Here's how the part is built. I have some questions about the finished solid (model axes, mm). Face numbers are marked on the shaded views. A direction names the side the tool comes from. Give positions to 0.01 mm unless a question says otherwise; leave off trailing zeros. Loops run counter-clockwise (first coordinate to the right, second up) from the corner with the lowest first, then second, coordinate; pieces in that order, holes last. Notation, with made-up numbers: (5, -4.5) - (42, -4.5) arc R14 cw to (42, 4.5) - close; hole circle Ø7 at (-40, 32.25). An arc over 180 degrees is marked (long way). Use one line per item in the form item = value.
from build123d import *

# Parameters (mm, degrees)
F0_R     = 1.795
F1_DEPTH = 3.1


with BuildPart() as f1:
    # F0 (on Front) → F1 (new body)
    with BuildSketch(Plane.XZ):
        with BuildLine():
            Line((-25.917618, 55.021677), (-33.917618, 50.898571))
            Line((-33.917618, 50.898571), (-33.917618, 30.898571))
            Line((-33.917618, 30.898571), (-26.205678, 16.406338))
            ThreePointArc((-26.205678, 16.406338), (-25.480558, 16.083714), (-24.99199, 16.709162))
            Line((-24.99199, 16.709162), (-24.99199, 34.125582))
            Line((-24.99199, 34.125582), (-28.417245, 37.768057))
            Line((-28.417245, 37.768057), (-28.417245, 42.768057))
            Line((-28.417245, 42.768057), (-22.746045, 37.125585))
            Line((-22.746045, 37.125585), (-22.746045, 24.125582))
            Line((-22.746045, 24.125582), (-20.271171, 21.650708))
            ThreePointArc((-20.271171, 21.650708), (-19.917618, 21.504262), (-19.564064, 21.650708))
            Line((-19.564064, 21.650708), (-17.089191, 24.125582))
            Line((-17.089191, 24.125582), (-17.089191, 37.125585))
            Line((-17.089191, 37.125585), (-11.41799, 42.768057))
            Line((-11.41799, 42.768057), (-11.41799, 37.768057))
            Line((-11.41799, 37.768057), (-14.843246, 34.125582))
            Line((-14.843246, 34.125582), (-14.843246, 16.690635))
            ThreePointArc((-14.843246, 16.690635), (-14.358181, 16.069672), (-13.638261, 16.389983))
            Line((-13.638261, 16.389983), (-5.917618, 30.898571))
            Line((-5.917618, 30.898571), (-5.917618, 50.898571))
            Line((-5.917618, 50.898571), (-13.917618, 55.021677))
            Line((-13.917618, 55.021677), (-25.917618, 55.021677))
        make_face()
        with Locations((-20.491593, 51.844455)):
            Circle(F0_R, mode=Mode.SUBTRACT)
    extrude(amount=F1_DEPTH)


solid = f1.part
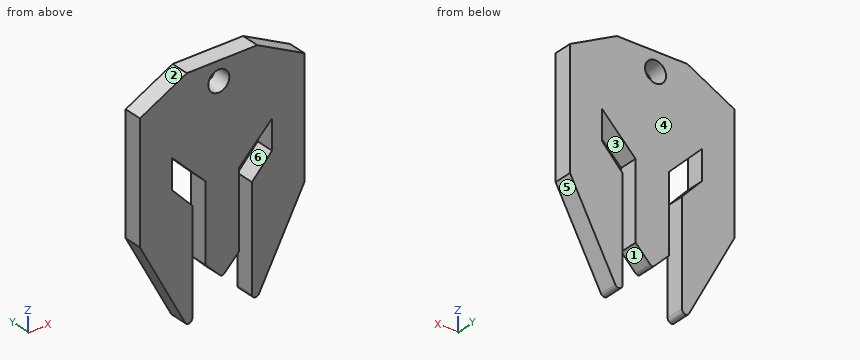
(1) For P1, Ø1, axis at x = -10.5, y = -1.5, coming from the -Z side; P2, Ø0.9, axis at y = -1.5, z = 29, coming from the +X side, each with a flat end and sliding along its axis, tell me the tip position at first contact or that it passes through.
Geometry says:
P1 = 21.35
P2 = -6.69
(2) For the marked faces 1, 2 and 3, which set-ups out of +Z, -Z, +X, -X, +Y, -Y let a thin tool reach every point of the face, with its end or its side?
Geometry says:
face_1 = -Z, +Y, -Y
face_2 = +Z, -X, +Y, -Y
face_3 = +Y, -Y
(3) If we section it at C-C (y = -0.5): List the corners of the cut face in (x, z) for me (3 decimals).
Geometry says:
outline = (-33.918, 30.899) - (-26.206, 16.406) arc R0.645 ccw to (-24.992, 16.709) - (-24.992, 34.126) - (-28.417, 37.768) - (-28.417, 42.768) - (-22.746, 37.126) - (-22.746, 24.126) - (-20.271, 21.651) arc R0.5 ccw to (-19.564, 21.651) - (-17.089, 24.126) - (-17.089, 37.126) - (-11.418, 42.768) - (-11.418, 37.768) - (-14.843, 34.126) - (-14.843, 16.691) arc R0.64 ccw to (-13.638, 16.39) - (-5.918, 30.899) - (-5.918, 50.899) - (-13.918, 55.022) - (-25.918, 55.022) - (-33.918, 50.899) - close; hole circle Ø3.59 at (-20.492, 51.844)
(4) If we section it at D-D (z = 25.5): List the corners of the cut face in (x, y) for me.
Geometry says:
outline = (-31.04, -3.1) - (-24.99, -3.1) - (-24.99, 0) - (-31.04, 0) - close; (-22.75, -3.1) - (-17.09, -3.1) - (-17.09, 0) - (-22.75, 0) - close; (-14.84, -3.1) - (-8.79, -3.1) - (-8.79, 0) - (-14.84, 0) - close
(5) If we section it at B-B (x = -27): List the corners of the cut face in (y, z) for me, plus the area to 4 significant figures.
Geometry says:
outline = (-3.1, 17.9) - (0, 17.9) - (0, 36.26) - (-3.1, 36.26) - close; (-3.1, 41.36) - (0, 41.36) - (0, 54.46) - (-3.1, 54.46) - close
area = 97.55 mm²
(6) If we section it at A-A (z = 32.5): List the corners of the cut face in (x, y) for me, plus the area to 3 significant figures.
Geometry says:
outline = (-33.92, -3.1) - (-24.99, -3.1) - (-24.99, 0) - (-33.92, 0) - close; (-22.75, -3.1) - (-17.09, -3.1) - (-17.09, 0) - (-22.75, 0) - close; (-14.84, -3.1) - (-5.92, -3.1) - (-5.92, 0) - (-14.84, 0) - close
area = 72.9 mm²
(7) Thinking about a two-plate mould opening in Z: for the marked faces 4, 5 and 6, which applies, pulls with the +Z half, pulls with the -Z half, needs draft (parallel to the pull), parting line crosses it, or undercut?
Geometry says:
face_4 = needs draft
face_5 = pulls with the -Z half
face_6 = undercut
(8) If I drill on probe 1 along X at (y, z) = (-0.5, 33); probe 2 along X at (y, z) = (-1.2, 27); probe 3 along X at (y, z) = (-0.8, 19.5), over which ranges is the centre line in solid material (lowest first)?
Geometry says:
probe_1 = -33.92 to -24.99, -22.75 to -17.09, -14.84 to -5.92
probe_2 = -31.84 to -24.99, -22.75 to -17.09, -14.84 to -7.99
probe_3 = -27.85 to -24.99, -14.84 to -11.98
